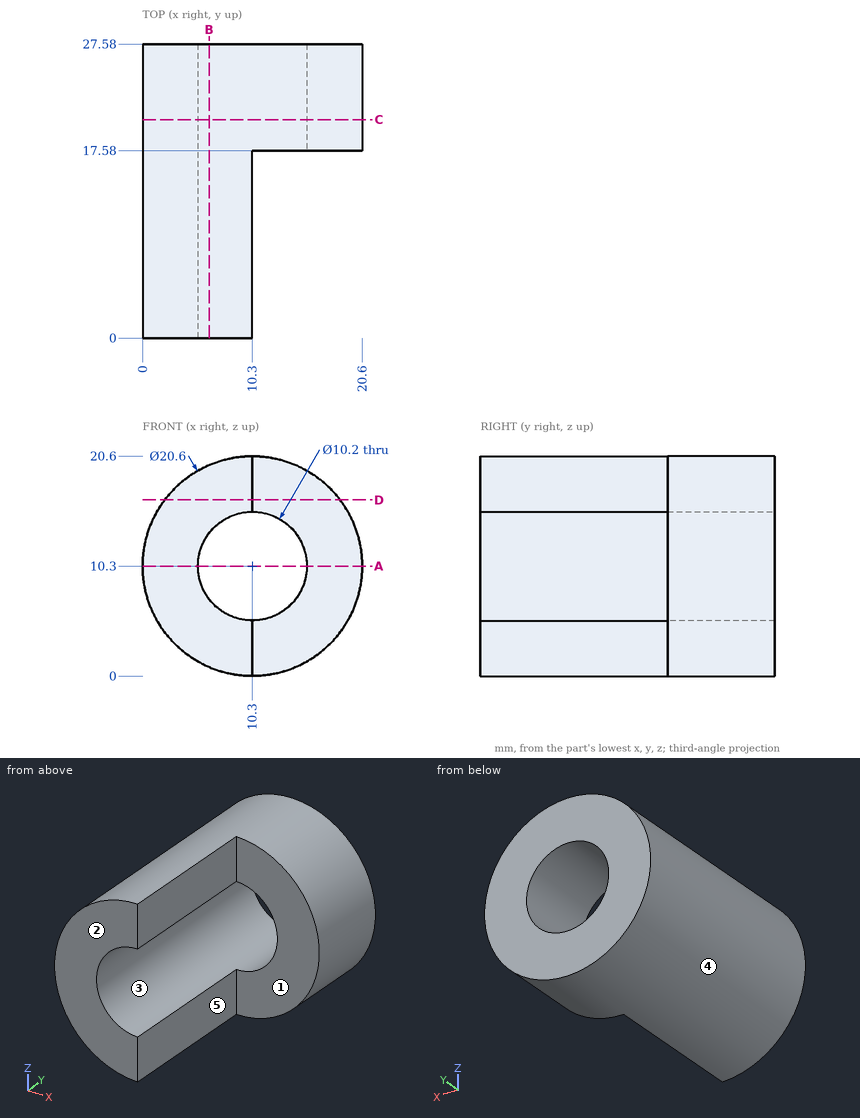
Print and shaded views of the part. All mm, measured from the part's lowest x, y and z. A direction names the side the tool comes from. Round coordinates to 2 decimals unless told otherwise and drop trailing zeros. Order: outer loops, then holes, each group sorted by start corner. A loop starts at its lowest first (then second) coordinate and runs counter-clockwise, first axis right, second up.
Q1. Slice it at D-D (z = 16.5). Write the cut outline in (x, y).
Q2. Slice it at A-A (z = 10.3). Write the cut outline in (x, y).
Q3. Slice it at C-C (y = 20.5). Write the cut outline in (x, z).
Q4. Two-plate mould, pull along Z, no slides. Class the marked faces 3, 4 and 5: pulls with the +Z half, pulls with the -Z half, needs draft (parallel to the pull), parting line crosses it, or undercut.
Q5. Wall check: L1, parallel to X at y = 18.5, z = 10.3; L2, parallel to Y at x = 19.75, z = 11.5; L3, parallel to X at y = 14, z = 10.3. Give the ranges that are in metal, low to high.
Q6. Which spindle directions (+Z, -Z, +X, -X, +Y, -Y) get a long thin tool onto all of the face, cutting with end or side? Do the marked faces 1 and 2. Say none if no direction does.
Q7. Drop flat-ended pins along their axis: pin 1 (2 mm diameter, centred on x = 6.5, z = 7.5, fed in from +Y); pin 2 (8 mm diameter, centred on x = 3, y = 10.5, fed in from +Z); pin 3 (5 mm diameter, centred on x = 18, y = 16, fed in from -Z); pin 4 (5.5 mm diameter, centred on y = 11.5, z = 18.5, fed in from +X). Give the stop position or say it passes through.
Q8. Slice it at B-B (x = 6.25). Write the cut outline in (y, z).
Results below:
1. outline: (2.08, 0) - (10.3, 0) - (10.3, 17.58) - (18.52, 17.58) - (18.52, 27.58) - (2.08, 27.58) - close
2. outline: (0, 0) - (5.2, 0) - (5.2, 27.58) - (0, 27.58) - close; (15.4, 17.58) - (20.6, 17.58) - (20.6, 27.58) - (15.4, 27.58) - close
3. outline: circle Ø20.6 at (10.3, 10.3); hole circle Ø10.2 at (10.3, 10.3)
4. face 3: undercut
4. face 4: parting line crosses it
4. face 5: needs draft
5. L1: x = 0 to 5.2, 15.4 to 20.6
5. L2: y = 17.58 to 27.58
5. L3: x = 0 to 5.2
6. face 1: +Z, -Z, +X, -Y
6. face 2: +Z, -Z, +X, -X, -Y
7. pin 1: stops at y = 27.58
7. pin 2: stops at z = 20.06
7. pin 3: stops at z = 1.76
7. pin 4: stops at x = 10.3
8. outline: (0, 0.83) - (27.58, 0.83) - (27.58, 7.2) - (0, 7.2) - close; (0, 13.4) - (27.58, 13.4) - (27.58, 19.77) - (0, 19.77) - close
